Read the model definition and answer for the solid it produces. Units are mm, in the model's axes. Coordinates: 2 decimals unless noted, no trailing zeros. Order: outer loops, then holes, each group sorted by start corner. A loop starts at its lowest first (then second) coordinate and runs counter-clockwise, first axis right, second up. Notation, with made-up numbers: M -19.75,37.5 L 15.25,37.5 A12 cw 15.25,51.5 Z; hole C 10,-20 d3. An arc over 180 degrees is marked long. Write each question's results on one line, items separated by ' | '.
```python
from build123d import *

# Parameters (mm, degrees)
SKETCH_1_R          = 3
EXTRUDE_1_DEPTH     = 3
EXTRUDE_START       = -3
SKETCH_2_R          = 3
EXTRUDE_2_DEPTH     = 3
EXTRUDE_4_DEPTH     = 3
FILLET_1_R          = 20
SKETCH_4_R          = 1
CUT_EXTRUDE_2_DEPTH = 134.77989332
SKETCH_5_R          = 1.5
CUT_EXTRUDE_3_DEPTH = 134.77989332
EXTRUDE_5_DEPTH     = 3
FILLET_2_R          = 2
FILLET_3_R          = 1


with BuildPart() as part:
    # 草图1 → 凸台-拉伸1 (new body)
    with BuildSketch(Plane(origin=(0, 0, 0), x_dir=(1, 0, 0), z_dir=(0, 1, 0))):
        with BuildLine():
            Line((0, 4), (70, 4))
            ThreePointArc((70, 4), (72.828427125, 2.828427125), (74, 0))
            Line((74, 0), (74, -10))
            ThreePointArc((74, -10), (61.386213612, -44.681924543), (29.439223407, -63.157132631))
            ThreePointArc((29.439223407, -63.157132631), (24.635207854, -84.826646437), (36.560916037, -103.546258569))
            ThreePointArc((36.560916037, -103.546258569), (37.297642861, -107.724444011), (33.119457419, -108.461170835))
            ThreePointArc((33.119457419, -108.461170835), (18.340459825, -82.982499926), (28.246224292, -55.243407089))
            ThreePointArc((28.246224292, -55.243407089), (55.321795077, -39.463169658), (66, -10))
            Line((66, -10), (66, -4))
            Line((66, -4), (0, -4))
            ThreePointArc((0, -4), (-4, 0), (0, 4))
        make_face()
        with Locations(Location((70, 0, 0), (0, 0, 270))):
            Circle(SKETCH_1_R, mode=Mode.SUBTRACT)
    extrude(amount=EXTRUDE_1_DEPTH)

    # 草图2 → 凸台-拉伸2 (add)
    with BuildSketch(Plane(origin=(0, 3, 0), x_dir=(1, 0, 0), z_dir=(0, 1, 0)).offset(EXTRUDE_START)):
        with BuildLine():
            Line((0, 4), (69.624462411, 7.490592201))
            ThreePointArc((69.624462411, 7.490592201), (73.786168915, -6.474173689), (63.65571123, 4))
            Line((63.65571123, 4), (0, 4))
        make_face()
        with Locations(Location((70, 0, 0), (0, 0, 270))):
            Circle(SKETCH_2_R, mode=Mode.SUBTRACT)
    extrude(amount=EXTRUDE_2_DEPTH)

    # 草图6 → 凸台-拉伸4 (add)
    with BuildSketch(Plane.XZ):
        with BuildLine():
            Line((70.702827497, -13.290378643), (71.760789381, -7.290378643))
            ThreePointArc((71.760789381, -7.290378643), (70.699822834, -7.467278487), (69.624462411, -7.490592201))
            Line((69.624462411, -7.490592201), (65.624462411, -7.290053937))
            Line((65.624462411, -7.290053937), (70.702827497, -13.290378643))
        make_face()
    extrude(amount=-EXTRUDE_4_DEPTH)

    # 圆角1
    fillet_1_edges = [part.edges().sort_by_distance(p)[0] for p in [
        (29.439223407, 1.5, 63.157132631),
        (28.246224292, 1.5, 55.243407089),
    ]]
    fillet(fillet_1_edges, radius=FILLET_1_R)

    # 草图4 → 切除-拉伸2 (cut, through all)
    with BuildSketch(Plane.XZ):
        with Locations(Location((62.705974414, 36, 0), (0, 0, 270))):
            Circle(SKETCH_4_R)
        with Locations(Location((34.840186728, 106.003714702, 0), (0, 0, 270))):
            Circle(SKETCH_4_R)
        with Locations(Location((0, 0, 0), (0, 0, 270))):
            Circle(SKETCH_4_R)
        with Locations(Location((69, -6.5, 0), (0, 0, 270))):
            Circle(SKETCH_4_R)
        with Locations(Location((12, 0, 0), (0, 0, 270))):
            Circle(SKETCH_4_R)
        with Locations(Location((24, 0, 0), (0, 0, 270))):
            Circle(SKETCH_4_R)
        with Locations(Location((36, 0, 0), (0, 0, 270))):
            Circle(SKETCH_4_R)
        with Locations(Location((35.04334559, 57.673267705, 0), (0, 0, 270))):
            Circle(SKETCH_4_R)
    extrude(amount=-CUT_EXTRUDE_2_DEPTH, mode=Mode.SUBTRACT)

    # 草图5 → 切除-拉伸3 (cut, through all)
    with BuildSketch(Plane(origin=(0, 3, 0), x_dir=(1, 0, 0), z_dir=(0, 1, 0))):
        with Locations(Location((48, 0, 0), (0, 0, 270))):
            Circle(SKETCH_5_R)
    extrude(amount=-CUT_EXTRUDE_3_DEPTH, mode=Mode.SUBTRACT)

    # 草图9 → 凸台-拉伸5 (add)
    with BuildSketch(Plane(origin=(0, 3, 0), x_dir=(1, 0, 0), z_dir=(0, 1, 0)).offset(EXTRUDE_START)):
        with BuildLine():
            Line((74, -10), (74, -6.873863542))
            ThreePointArc((74, -6.873863542), (74.209430585, -7.486235978), (74.75, -7.842109379))
            ThreePointArc((74.75, -7.842109379), (75.499999137, -8.811669003), (74.747455001, -9.779254603))
            ThreePointArc((74.747455001, -9.779254603), (74.20933726, -10.129384674), (73.995002571, -10.734547803))
            ThreePointArc((73.995002571, -10.734547803), (73.998750628, -10.367282401), (74, -10))
        make_face()
    extrude(amount=EXTRUDE_5_DEPTH)

    # 圆角2
    fillet_2_edges = [part.edges().sort_by_distance(p)[0] for p in [
        (0, 1.5, -4),
        (66, 1.5, 6.34428877),
        (63.65571123, 1.5, 4),
        (65.624462411, 1.5, -7.290053937),
        (71.760789381, 1.5, -7.290378643),
    ]]
    fillet(fillet_2_edges, radius=FILLET_2_R)

    # 圆角3
    fillet_3_edges = [part.edges().sort_by_distance(p)[0] for p in [
        (70.702827497, 1.5, -13.290378643),
        (74, 1.5, 6.34428877),
    ]]
    fillet(fillet_3_edges, radius=FILLET_3_R - 0.0001)  # a hair under: the kernel refuses the full size


solid = part.part
```
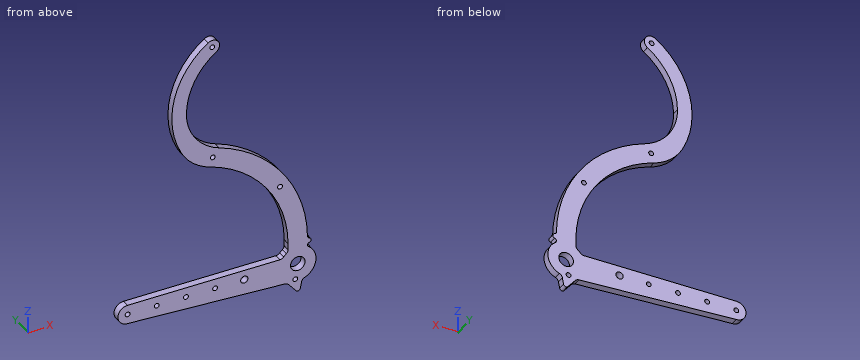
(1) Straight lines are drawn through the part: line 1 (Z direction, x = 49, y = 1.3); line 2 (Z direction, x = 35.5, y = 2.25); line 3 (Z direction, x = 55, y = 1). For each, find the intervals that lie inside material, in ascending order.
Conclusion:
line 1: -6.46 to -1.12, 1.12 to 4, 45.7 to 55.54 | line 2: -5.78 to -0.87, 0.87 to 4, 53.3 to 56.78, 58.56 to 61.91, 102.77 to 105.25, 106.76 to 108.93 | line 3: -6.76 to 4, 39.84 to 51.12
(2) The part is cut by section C-C, the plane x = 9. Write down the section's boundary in (y, z), then the cut area to 3 significant figures.
Conclusion:
outline: M 0,-4.45 L 3,-4.45 L 3,4 L 0,4 Z | area: 25.4 mm²
(3) The part is cut by section A-A, the plane x = 29.5. Count the separate pieces of the cut face and the enclosed holes in it, then the cut area to 3 significant figures.
Conclusion:
separate pieces: 3 | enclosed holes: 0 | area: 87.2 mm²
(4) Given pin 1 (2.5 mm diameter, centred on x = 48, z = 0, fed in from -Y); pin 2 (0.8 mm diameter, centred on y = 1.5, z = 8, fed in from -X); pin 3 (1 mm diameter, centred on x = 40.5, y = 1, fed in from -Z); pin 4 (1 mm diameter, centred on x = 6, y = 2, fed in from +Z), each flat-ended and moving along its own axis, determine where each tip first touches the part or whether it passes through.
Conclusion:
pin 1: through | pin 2: x = 66 | pin 3: z = -6.06 | pin 4: z = 4
